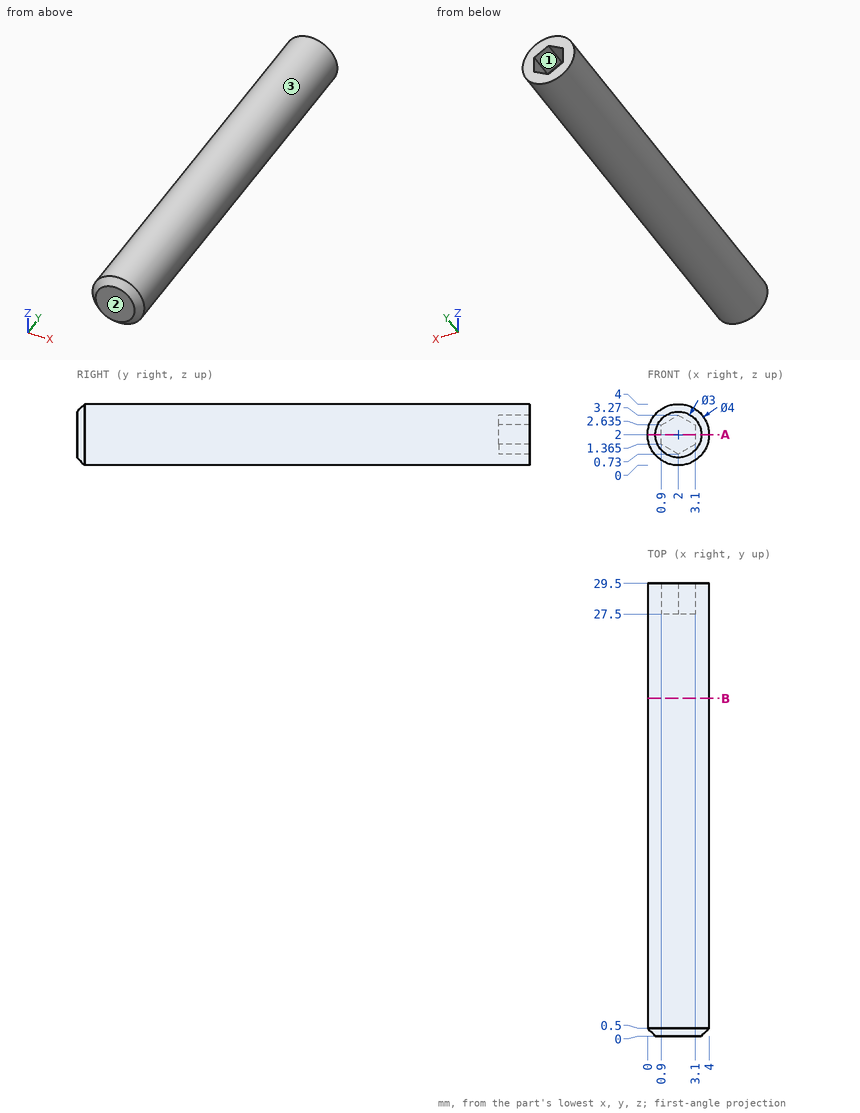
For this review, use the dimensioned drawing (mm, ordinates from the lowest corner) and the shaded views. Coordinates: 2 decimals unless noted, no trailing zeros. Write each loop counter-clockwise with the first axis right and the second up, starting at its lowest first coordinate (ties: lowest second). Pieces come first, ordered by that corner, then holes. Notation, with made-up numbers: (-24, -10) -> (12, -10) arc R23 ccw to (12, 28) -> close; hole circle Ø11 at (2.25, 39). An arc over 180 degrees is marked (long way). Put each result on its own line as item: value.
Q1. Clearance check with flat-ended pins moving along their axes: pin 1 Ø2 at (x, z) = (3.5, 2) entering from -Y; pin 2 Ø1.5 at (y, z) = (25, 3.5) entering from -X; pin 3 Ø0.7 at (x, z) = (2, 2) entering from +Y. State where each tip first meets the part, or that it passes through.
From the geometry:
pin 1: stops at y = 0
pin 2: stops at x = 0.15
pin 3: stops at y = 27.5
Q2. Take a section at A-A, the plane z = 2. State the section outline as (x, y) points, then the cut area to 3 significant figures.
From the geometry:
outline: (0, 0.5) -> (0.5, 0) -> (3.5, 0) -> (4, 0.5) -> (4, 29.5) -> (3.1, 29.5) -> (3.1, 27.5) -> (0.9, 27.5) -> (0.9, 29.5) -> (0, 29.5) -> close
area: 113 mm2
Q3. Wall thickness on L1, parallel to Y at x = 1.55, z = 1.1; L2, parallel to Z at x = 1.9, y = 1.5; L3, parallel to X at y = 5.25, z = 2.15: over which ranges is each line inside the solid? List them lowest first.
From the geometry:
L1: y = 0 to 27.5
L2: z = 0 to 4
L3: x = 0.01 to 3.99
Q4. The part is to be moulded in two halves that separate along X. For the marked faces 1, 2 and 3, say which applies: +X half, -X half, draft (parallel to the pull), parting line (faces both ways), or undercut.
From the geometry:
face 1: undercut
face 2: draft
face 3: parting line
Q5. Take a section at B-B, the plane y = 22. State the section outline as (x, z) points.
From the geometry:
outline: circle Ø4 at (2, 2)
